For this review, use the dimensioned drawing (mm, ordinates from the lowest corner) and the shaded views. A direction names the side the tool comes from. Round coordinates to 2 decimals unless told otherwise and drop trailing zeros. Loops run counter-clockwise (first coordinate to the right, second up) from the corner with the lowest first, then second, coordinate; pieces in that order, holes last. Notation, with made-up numbers: (42, -20) -> (70, -20) arc R25 ccw to (70, 12) -> close; hole circle Ø9 at (-12.5, 46.5). An arc over 180 degrees is marked (long way). Write each question's results on one line, items separated by ' | '. Start each with the question number.
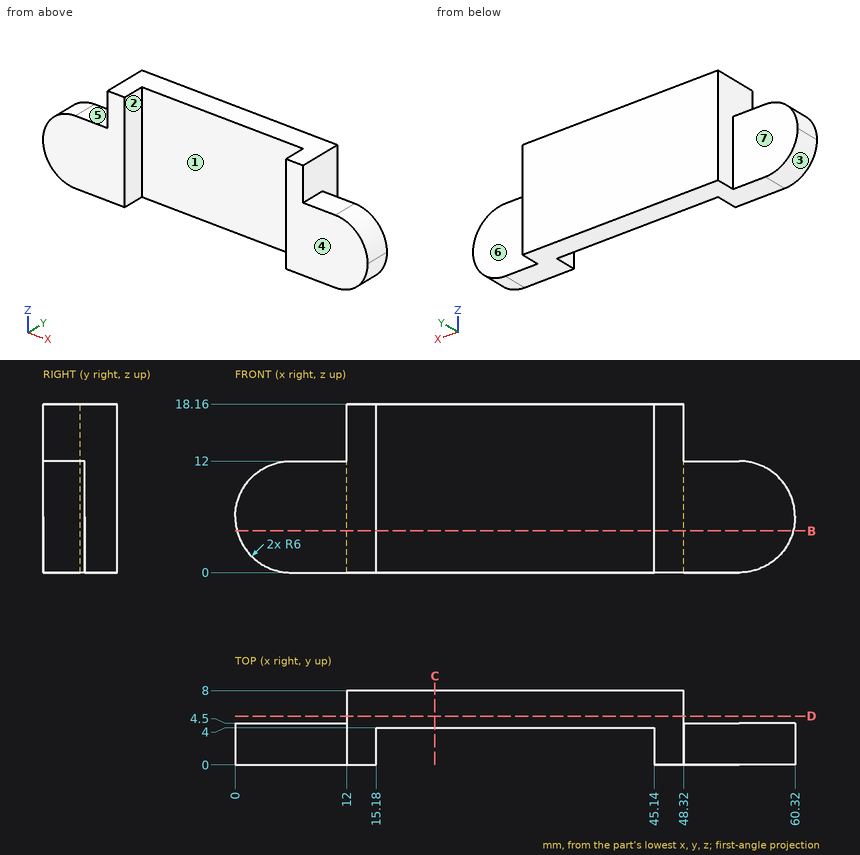
1) The part is to be moulded in two halves that separate along X. For the marked faces 1, 2, 3 and 4, say which applies: +X half, -X half, draft (parallel to the pull), parting line (faces both ways), or undercut.
2) To check wall thickness, follow line 1 (X direction, y = 1.75, z = 12.75); line 2 (Z direction, x = 53, y = 3.5); line 3 (Y direction, x = 8, z = 11.5). State the ranges of each line that lie inside material, in increasing order. Write a range as from..to.
3) Take a section at B-B (z = 4.5). Write out the cut boundary in (x, y).
4) Take a section at C-C (x = 21.5). Write out the cut boundary in (y, z).
5) For the marked faces 5, 6 and 7, list the 3-axis set-ups (+Z, -Z, +X, -X, +Y, -Y) from which the entire face can be reached by the end or side of a thin tool; tool diameter is ignored.
6) Take a section at D-D (y = 5.25). Write out the cut boundary in (x, z), plus the area to 3 significant figures.
7) Insertion check: pin 1 (9.5 mm diameter, centred on x = 5, z = 5, fed in from +Y); pin 2 (6 mm diameter, centred on x = 25.5, z = 16, fed in from -Y); pin 3 (1.5 mm diameter, centred on y = 2, z = 14.5, fed in from +X). Each pin has a flat end and moves straight along its axis. Give the tip position at first contact, or say it passes through.
Geometry check:
1) face 1: undercut | face 2: undercut | face 3: -X half | face 4: draft
2) line 1: x = 12..15.18, 45.14..48.32 | line 2: z = 0..12 | line 3: y = 0..4.5
3) outline: (0.19, 0) -> (15.18, 0) -> (15.18, 4) -> (45.14, 4) -> (45.14, 0) -> (60.13, 0) -> (60.13, 4.5) -> (48.32, 4.5) -> (48.32, 8) -> (12, 8) -> (12, 4.5) -> (0.19, 4.5) -> close
4) outline: (4, 0) -> (8, 0) -> (8, 18.16) -> (4, 18.16) -> close
5) face 5: +Z, -X, +Y, -Y | face 6: +Z, -Z, +X, +Y | face 7: +Z, -Z, -X, +Y
6) outline: (12, 0) -> (48.32, 0) -> (48.32, 18.16) -> (12, 18.16) -> close | area: 660 mm^2
7) pin 1: stops at y = 4.5 | pin 2: stops at y = 4 | pin 3: stops at x = 48.32
